Geometry check sheet. Reference: the model listing, model coordinates, mm. A direction names the side the tool comes from. Give positions to 0.01 mm unless a question says otherwise; leave off trailing zeros. Order: outer loops, then holes, each group sorted by start corner. A loop starts at its lowest first (then second) coordinate and runs counter-clockwise, first axis right, second up. Notation, with made-up numbers: M 47.5,19 L 78.5,19 A18 cw 78.5,54 Z; hole C 27.25,33 d9. An arc over 180 degrees is marked long. Put each result on its own line as item: value. Start each with the question number.
Q1. Material ranges on L1, parallel to Y at x = -81.5, z = 92; L2, parallel to Y at x = -90, z = 129.5; L3, parallel to X at y = 84, z = 79, recorded low to high.
Q2. Section check A-A on x = -53. Record the cut outline in (y, z), then the cut area to 3 significant figures.
Q3. Section check C-C on y = 136.5. Record the cut outline in (x, z), then the cut area to 3 significant figures.
Q4. Mould release check, pull along Y, two halves, no side actions. Record for faces 1 (the flat face through (-86, 20, 83)), 2 (the flat face through (0, 111, 131)), 3 (the flat face through (-86, 18, 83)): +Y half, -Y half, draft (parallel to the pull), parting line (faces both ways), or undercut.
Q5. Section check B-B on z = 139. Record the cut outline in (x, y).
Q6. Access from +Z, -Z, +X, -X, +Y, -Y to the whole of each face (thin tool, end or side, straight path). Record for faces 4 (the flat face through (-111, 0, 131)), 5 (the cylindrical face through (-69.93, 18.99, 71.48)).
Q7. Go/stop test with flat-tipped pins: pin 1 (5 mm diameter, centred on x = -27.76, z = 105.54, fed in from +Y); pin 2 (10 mm diameter, centred on y = 40, z = 109, fed in from -X); pin 3 (2 mm diameter, centred on y = 31, z = 110.5, fed in from +X). Record where each tip stops, or that it passes through.
Autodesk Inventor part; units mm, degrees
ref_plane "YZ Plane" through (0, 0, 0) normal (1, 0, 0) x (0, 1, 0)
ref_plane "XZ Plane" through (0, 0, 0) normal (0, 1, 0) x (-1, 0, 0)
ref_plane "XY Plane" through (0, 0, 0) normal (0, 0, 1) x (1, 0, 0)
sketch "Sketch1" plane through (0, 0, 0) normal (0, 1, 0) x (-1, 0, 0)
  arc A0 (172, 0) -> (0, 172) centre (0, 0) ccw
  line L0 (0, 172) -> (0, 0)
  line L1 (172, 0) -> (0, 0)
revolve "Revolution1" add sketch "Sketch1" angle 90 about axis through (0, 0, 172) along (0, 0, -1)
sketch "Sketch2" plane through (-172, 0, 0) normal (0, -1, 0) x (1, 0, 0)
  arc A0 (172, 170) -> (2, 0) centre (172, 0) ccw
  line L0 (172, 0) -> (172, 172)
  line L1 (172, 0) -> (2, 0)
  line L2 (172, 0) -> (172, 170)
revolve "Revolution2" cut sketch "Sketch2" angle 90 about axis through (0, 0, 0) along (0, 0, -1)
sketch "Sketch3" plane through (0, 0, 0) normal (1, 0, 0) x (0, -0.7071068, -0.7071068)
  arc A0 (-121.6224, 121.6224) -> (-121.6224, -121.6224) centre (0, 0) ccw
  arc A1 (-120.2082, 120.2082) -> (-120.2082, -120.2082) centre (0, 0) ccw
  line L0 (-121.6224, -121.6224) -> (-101.6224, -121.6224) construction
  line L1 (0, 0) -> (-121.6224, 121.6224)
  line L2 (0, 0) -> (-14.1421, 14.1421)
  line L3 (-84.8528, -56.5685) -> (-133.5155, -105.2312)
  line L4 (-84.8528, -56.5685) -> (-83.4386, -57.9828)
  line L5 (-83.4386, -57.9828) -> (-132.2603, -106.8045)
  point P0 (-134.7537, -103.641)
  dimension "d49" = 2
revolve "Revolution3" add sketch "Sketch3" angle 90 about axis through (0, 0, 0) along (0, -1, 0)
sketch "Sketch7" plane through (0, 20, 168.8194) normal (0, 1, 0) x (1, 0, 0)
  circle A0 centre (-27.763, 63.2747) radius 1.5
  circle A1 centre (-77.0746, 91.7448) radius 1.5
  circle A2 centre (-105.5447, 141.0564) radius 1.5
  line L0 (-77.7817, 91.0377) -> (-77.0746, 91.7448)
  line L1 (-77.7817, 91.0377) -> (-76.7817, 91.0377) construction
  dimension "d57" = 3
  dimension "d58" = 3
  dimension "d59" = 3
  dimension "d62" = 1
  dimension "d63" = 45
extrude "Extrusion4" cut sketch "Sketch7" against normal blind 10
properties part number "shell" material "Glass"
Results found:
1. L1: y = 18 to 20, 117.45 to 120.32
1. L2: y = 18 to 20, 63.48 to 68.66
1. L3: x = -127.62 to -124.91
2. outline: M 0,161.53 A161.53 cw 18,160.52 L 18,84.8 L 20,84.8 L 20,160.28 A161.53 cw 161.53,0 L 163.63,0 A163.63 ccw 0,163.63 Z
2. area: 688 mm^2
3. outline: M -104.65,0 L -101.33,0 A101.33 cw 0,101.33 L 0,104.65 A104.65 ccw Z
3. area: 537 mm^2
4. face 1: undercut
4. face 2: draft
4. face 3: -Y half
5. outline: M -101.31,0 L -97.87,0 A97.87 cw -96.2,18 L 0,18 L 0,20 L -95.81,20 A97.87 cw 0,97.87 L 0,101.31 A101.31 ccw Z
6. face 4: +Z, -Z, +X, -X, -Y
6. face 5: -Z, +X, -Y
7. pin 1: stops at y = 134.96
7. pin 2: stops at x = -131.3
7. pin 3: stops at x = -124.49
